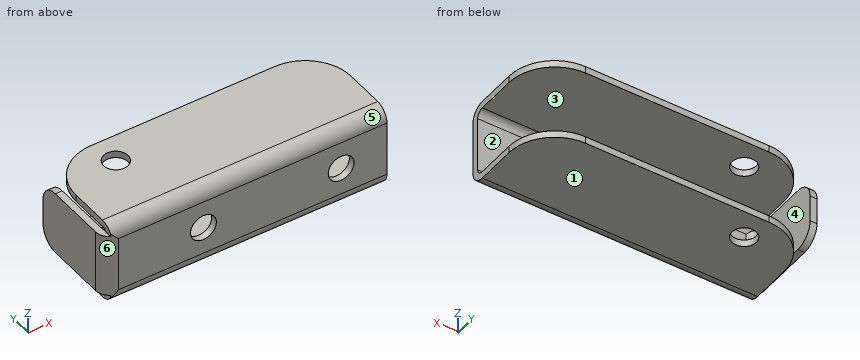
```python
from build123d import *

# Parameters (mm, degrees)
SKETCH1_W           = 78.105
SKETCH1_H           = 22.86
BOSS_EXTRUDE1_DEPTH = 1.905
SKETCH2_W           = 76.2
SKETCH2_H           = 1.905
BOSS_EXTRUDE2_DEPTH = 25.527
SKETCH5_W           = 1.905
SKETCH5_H           = 17.526
BOSS_EXTRUDE6_DEPTH = 23.495
SKETCH6_W           = 1.905
SKETCH6_H           = 2.667
CUT_EXTRUDE2_DEPTH  = 25.4
SKETCH7_R           = 3.5687
CUT_EXTRUDE3_DEPTH  = 25.4
SKETCH8_R           = 3.3655
CUT_EXTRUDE4_DEPTH  = 25.4
FILLET1_R           = 12.7
FILLET2_R           = 5.08
FILLET3_R           = 3.81
FILLET4_R           = 1.905
FILLET5_R           = 3.81
FILLET6_START       = 1.905
FILLET6_DEPTH       = 76.2


with BuildPart() as part:
    # Sketch1 → Boss-Extrude1 (new body)
    with BuildSketch(Plane(origin=(0, 0, 0), x_dir=(1, 0, 0), z_dir=(0, 1, 0))):
        with Locations((39.0525, 0)):
            Rectangle(SKETCH1_W, SKETCH1_H)
    extrude(amount=BOSS_EXTRUDE1_DEPTH)

    # Sketch2 → Boss-Extrude2 (add)
    with BuildSketch(Plane(origin=(0, 1.905, 0), x_dir=(1, 0, 0), z_dir=(0, 1, 0))):
        with Locations((40.005, -10.4775)):
            Rectangle(SKETCH2_W, SKETCH2_H)
        with Locations((40.005, 10.4775)):
            Rectangle(SKETCH2_W, SKETCH2_H)
    extrude(amount=BOSS_EXTRUDE2_DEPTH)

    # Sketch5 → Boss-Extrude6 (add)
    with BuildSketch(Plane(origin=(0, 1.905, 0), x_dir=(1, 0, 0), z_dir=(0, 1, 0))):
        with Locations((0.9525, 0)):
            Rectangle(SKETCH5_W, SKETCH5_H)
    extrude(amount=BOSS_EXTRUDE6_DEPTH)

    # Sketch6 → Cut-Extrude2 (cut)
    with BuildSketch(Plane(origin=(0, 1.905, 0), x_dir=(1, 0, 0), z_dir=(0, 1, 0))):
        with Locations((0.9525, -10.0965)):
            Rectangle(SKETCH6_W, SKETCH6_H)
        with Locations((0.9525, 10.0965)):
            Rectangle(SKETCH6_W, SKETCH6_H)
    extrude(amount=-CUT_EXTRUDE2_DEPTH, mode=Mode.SUBTRACT)

    # Sketch7 → Cut-Extrude3 (cut)
    with BuildSketch(Plane(origin=(0, 1.905, 0), x_dir=(1, 0, 0), z_dir=(0, 1, 0))):
        with Locations(Location((65.405, 0, 0), (0, 0, 270))):
            Circle(SKETCH7_R)
        with Locations(Location((27.305, 0, 0), (0, 0, 270))):
            Circle(SKETCH7_R)
    extrude(amount=-CUT_EXTRUDE3_DEPTH, mode=Mode.SUBTRACT)

    # Sketch8 → Cut-Extrude4 (cut)
    with BuildSketch(Plane.XY.offset(11.43)):
        with Locations((16.383, 19.812)):
            Circle(SKETCH8_R)
    extrude(amount=-CUT_EXTRUDE4_DEPTH, mode=Mode.SUBTRACT)

    # Fillet1
    fillet1_edges = [part.edges().sort_by_distance(p)[0] for p in [
        (78.105, 27.432, 10.4775),
        (1.905, 27.432, 10.4775),
        (1.905, 27.432, -10.4775),
        (78.105, 27.432, -10.4775),
    ]]
    fillet(fillet1_edges, radius=FILLET1_R)

    # Fillet2
    fillet2_edges = [part.edges().sort_by_distance(p)[0] for p in [
        (0.9525, 25.4, -8.763),
        (0.9525, 25.4, 8.763),
    ]]
    fillet(fillet2_edges, radius=FILLET2_R)

    # Fillet3
    fillet3_edges = [part.edges().sort_by_distance(p)[0] for p in [
        (0, 0, 0),
    ]]
    fillet(fillet3_edges, radius=FILLET3_R)

    # Fillet4
    fillet4_edges = [part.edges().sort_by_distance(p)[0] for p in [
        (1.905, 1.905, 0),
    ]]
    fillet(fillet4_edges, radius=FILLET4_R)

    # Fillet5
    # the kernel refuses this fillet: 3.81 mm, written as the material it takes off along each edge
    with BuildSketch(Plane(origin=(-5.715, 0, -11.43), x_dir=(0, 0, 1), z_dir=(1, 0, 0))) as fillet5_piece_1:
        with BuildLine():
            CenterArc((FILLET5_R, -FILLET5_R), FILLET5_R, 90, 90)
            Line((0, -FILLET5_R), (0, 0))
            Line((0, 0), (FILLET5_R, 0))
        make_face()
    extrude(amount=93.345, mode=Mode.SUBTRACT)
    with BuildSketch(Plane(origin=(87.63, 0, 11.43), x_dir=(0, 1, 0), z_dir=(-1, 0, 0))) as fillet5_piece_2:
        with BuildLine():
            CenterArc((FILLET5_R, FILLET5_R), FILLET5_R, 180, 90)
            Line((0, FILLET5_R), (0, 0))
            Line((0, 0), (FILLET5_R, 0))
        make_face()
    extrude(amount=93.345, mode=Mode.SUBTRACT)

    # Fillet6: read off the stored shape, not the designer's step
    # Fillet6 outline → Fillet6 (add)
    with BuildSketch(Plane.YZ.offset(FILLET6_START)):
        with BuildLine():
            Line((1.905, -7.62), (1.905, -9.525))
            Line((1.905, -9.525), (3.81, -9.525))
            ThreePointArc((3.81, -9.525), (2.462961582, -8.967038418), (1.905, -7.62))
        make_face()
        with BuildLine():
            Line((3.81, 9.525), (1.905, 9.525))
            Line((1.905, 9.525), (1.905, 7.62))
            ThreePointArc((1.905, 7.62), (2.462961582, 8.967038418), (3.81, 9.525))
        make_face()
    extrude(amount=FILLET6_DEPTH)


solid = part.part
```
Input: part model. Units: mm. Frame: model coordinates. Face numbers are marked on the shaded views. A direction names the side the tool comes from. Coordinates: 2 decimals unless noted, no trailing zeros. Loops run counter-clockwise (first coordinate to the right, second up) from the corner with the lowest first, then second, coordinate; pieces in that order, holes last.
Q1. Contact query for flat-ended pins moving along their axis: pin 1 (2 mm diameter, centred on x = 1, y = 11, fed in from -Z); pin 2 (3 mm diameter, centred on y = 8.5, z = -10.5, fed in from -X) (3 decimals); pin 3 (5 mm diameter, centred on y = 22.5, z = 1, fed in from +X) (3 decimals); pin 4 (0.6 mm diameter, centred on x = 1.5, z = 0.5, fed in from +Y). Output: stop coordinate, or through.
Results are:
pin 1: stops at z = -11.43
pin 2: stops at x = 1.905
pin 3: stops at x = 1.905
pin 4: stops at y = 25.4
Q2. Section A-A, the plane y = 11.25. Return the cut outline in (x, z) (3 decimals).
Results are:
outline: (0, -8.763) - (1.905, -8.763) - (1.905, 8.763) - (0, 8.763) - close; (1.905, -11.43) - (78.105, -11.43) - (78.105, -9.525) - (1.905, -9.525) - close; (1.905, 9.525) - (78.105, 9.525) - (78.105, 11.43) - (1.905, 11.43) - close
Q3. Set-up query: the marked faces 1, 2 and 3. Return all of +Z, -Z, +X, -X, +Y, -Y with unobstructed straight access to the full face (end or side cutting, diameter ignored); none if empty.
Results are:
face 1: -Z, +X, -X, +Y, -Y
face 2: +X, +Y
face 3: +X, -X, +Y
Q4. Section C-C, the plane x = 54. Return the cut outline in (y, z) (3 decimals).
Results are:
outline: (0, -7.62) arc R3.81 ccw to (3.81, -11.43) - (27.432, -11.43) - (27.432, -9.525) - (3.81, -9.525) arc R1.905 cw to (1.905, -7.62) - (1.905, 7.62) arc R1.905 cw to (3.81, 9.525) - (27.432, 9.525) - (27.432, 11.43) - (3.81, 11.43) arc R3.81 ccw to (0, 7.62) - close
Q5. Section B-B, the plane z = 0. Return the cut outline in (x, y) (3 decimals).
Results are:
outline: (0, 3.81) arc R3.81 ccw to (3.81, 0) - (23.736, 0) - (23.736, 1.905) - (3.81, 1.905) arc R1.905 cw to (1.905, 3.81) - (1.905, 25.4) - (0, 25.4) - close; (30.874, 0) - (61.836, 0) - (61.836, 1.905) - (30.874, 1.905) - close; (68.974, 0) - (78.105, 0) - (78.105, 1.905) - (68.974, 1.905) - close
Q6. Line query: line 1 along Z through (x, y) = (11.5, 10.25) (3 decimals); line 2 along X through (y, z) = (0.45, 0) (3 decimals); line 3 along Y through (x, z) = (17.5, -1.75) (3 decimals). Output: solid intervals per line, ascending.
Results are:
line 1: z = -11.43 to -9.525, 9.525 to 11.43
line 2: x = 2.014 to 23.736, 30.874 to 61.836, 68.974 to 78.105
line 3: y = 0 to 1.905
Q7. Section D-D, the plane x = 63.5. Return the cut outline in (y, z) (3 decimals), and give its area (3 significant figures).
Results are:
outline: (0, -7.62) arc R3.81 ccw to (3.81, -11.43) - (27.432, -11.43) - (27.432, -9.525) - (3.81, -9.525) arc R1.905 cw to (1.905, -7.62) - (1.905, -3.018) - (0, -3.018) - close; (0, 3.018) - (1.905, 3.018) - (1.905, 7.62) arc R1.905 cw to (3.81, 9.525) - (27.432, 9.525) - (27.432, 11.43) - (3.81, 11.43) arc R3.81 ccw to (0, 7.62) - close
area: 125 mm2
Q8. Mould query, pull axis Z, two halves, no side actions, for the marked faces 4, 5 and 6. Classes: +Z half, -Z half, draft (parallel to the pull), parting line (faces both ways), or undercut.
Results are:
face 4: undercut
face 5: +Z half
face 6: draft
